```python
from build123d import *

# Parameters (mm, degrees)
SKETCH1_W           = 20
SKETCH1_H           = 25
BOSS_EXTRUDE1_DEPTH = 4
SKETCH2_W           = 3
SKETCH2_H           = 12
BOSS_EXTRUDE2_DEPTH = 12
SKETCH3_R           = 2.25
CUT_EXTRUDE1_DEPTH  = 18.5
CHAMFER1_SIZE       = 0.75


with BuildPart() as part:
    # Sketch1 → Boss-Extrude1 (new body)
    with BuildSketch(Plane(origin=(0, 0, 0), x_dir=(0, 0, -1), z_dir=(1, 0, 0))):
        with Locations((10, -12.5)):
            Rectangle(SKETCH1_W, SKETCH1_H)
    extrude(amount=BOSS_EXTRUDE1_DEPTH)

    # Sketch2 → Boss-Extrude2 (add)
    with BuildSketch(Plane.ZY):
        with Locations((-10, -12.5)):
            Rectangle(SKETCH2_W, SKETCH2_H)
        with Locations((-4, -12.5)):
            Rectangle(SKETCH2_W, SKETCH2_H)
        with Locations((-16, -12.5)):
            Rectangle(SKETCH2_W, SKETCH2_H)
    extrude(amount=BOSS_EXTRUDE2_DEPTH)

    # Sketch3 → Cut-Extrude1 (cut, through all)
    with BuildSketch(Plane(origin=(0, 0, -17.5), x_dir=(-1, 0, 0), z_dir=(0, 0, -1))):
        with Locations((6, -12.5)):
            Circle(SKETCH3_R)
        with BuildLine():
            Line((12, -6.5), (6, -6.5))
            ThreePointArc((6, -6.5), (10.242640687, -8.257359313), (12, -12.5))
            Line((12, -12.5), (12, -6.5))
        make_face()
        with BuildLine():
            Line((12, -18.5), (12, -12.5))
            ThreePointArc((12, -12.5), (10.242640687, -16.742640687), (6, -18.5))
            Line((6, -18.5), (12, -18.5))
        make_face()
    extrude(amount=-CUT_EXTRUDE1_DEPTH, mode=Mode.SUBTRACT)

    # Chamfer1
    chamfer1_edges = [part.edges().sort_by_distance(p)[0] for p in [
        (-3.75, -12.5, -17.5),
    ]]
    chamfer(chamfer1_edges, length=CHAMFER1_SIZE)


solid = part.part
```
Geometry check sheet. Reference: the model listing, model coordinates, mm. A direction names the side the tool comes from. Coordinates: 2 decimals unless noted, no trailing zeros. Order: outer loops, then holes, each group sorted by start corner. A loop starts at its lowest first (then second) coordinate and runs counter-clockwise, first axis right, second up. Notation, with made-up numbers: (-9, 65.5) - (13, 65.5) arc R31 cw to (13, 93.5) - close; hole circle Ø5 at (53, -15.75). An arc over 180 degrees is marked (long way). Answer as a JSON object with one key per item and string values. Group by question number.
Item 1: Draft check along Z on faces 4 (the face through (0, -12, -12)), 5 (the face through (-3, -6.5, -4)), 6 (the face through (2, -13, 0)). Enter one of: +Z half, -Z half, draft (parallel to the pull), parting line (faces both ways), or undercut.
Item 2: Sectioned sample at D-D, the plane z = -2. Record the cut outline in (x, y), and give its area (3 significant figures).
Item 3: Tool access check on faces 1 (the face through (-3, -11, -17.5)), 2 (the face through (-3, -13, -8.5)), 3 (the face through (-3, -18.5, -10)). Record the directions out of +Z, -Z, +X, -X, +Y, -Y that give a thin tool (end or side, any length) a straight path to the whole face; none if there is none.
Item 4: Sectioned sample at A-A, the plane x = -10.75. Record the cut outline in (y, z).
Item 5: Sectioned sample at C-C, the plane y = -22.5. Record the cut outline in (x, z).
Item 6: Scan lines: probe 1 along Z at (x, y) = (-9.5, -11.25); probe 2 along Y at (x, z) = (-6, -15.3); probe 3 along X at (y, z) = (-7.5, -2). Record each from-to range of solid material in increasing order.
Item 7: Depth check by flat-ended pin: pin 1 Ø2.5 at (x, y) = (-6, -12.5) entering from +Z; pin 2 Ø9.5 at (x, y) = (-4.5, -15) entering from -Z; pin 3 Ø1.5 at (x, z) = (-1.5, -15.5) entering from +Y; pin 4 Ø0.9 at (x, z) = (-2, -4) entering from -Y. Enter the tip coordinate at first touch or a pass-through.
Item 8: Sectioned sample at B-B, the plane z = -10.25. Record the cut outline in (x, y).
Resolved:
{
 "1": {"face 4": "undercut", "face 5": "draft", "face 6": "+Z half"},
 "2": {"outline": "(0, -25) - (4, -25) - (4, 0) - (0, 0) - close", "area": "100 mm^2"},
 "3": {"face 1": "-Z, -X, +Y, -Y", "face 2": "-X, +Y, -Y", "face 3": "+Z, -Z, -X, -Y"},
 "4": {"outline": "(-16.17, -17.5) - (-8.83, -17.5) - (-8.83, -14.5) - (-16.17, -14.5) - close; (-16.17, -11.5) - (-8.83, -11.5) - (-8.83, -8.5) - (-16.17, -8.5) - close; (-16.17, -5.5) - (-8.83, -5.5) - (-8.83, -2.5) - (-16.17, -2.5) - close"},
 "5": {"outline": "(0, -20) - (4, -20) - (4, 0) - (0, 0) - close"},
 "6": {"probe 1": "-17.5 to -14.5, -11.5 to -8.5, -5.5 to -2.5", "probe 2": "-18.5 to -14.75, -10.25 to -6.5", "probe 3": "0 to 4"},
 "7": {"pin 1": "through", "pin 2": "z = -20", "pin 3": "y = -6.5", "pin 4": "y = -18.5"},
 "8": {"outline": "(-6, -18.5) - (0, -18.5) - (0, -25) - (4, -25) - (4, 0) - (0, 0) - (0, -6.5) - (-6, -6.5) arc R6 ccw to start; hole circle Ø4.5 at (-6, -12.5)"}
}
